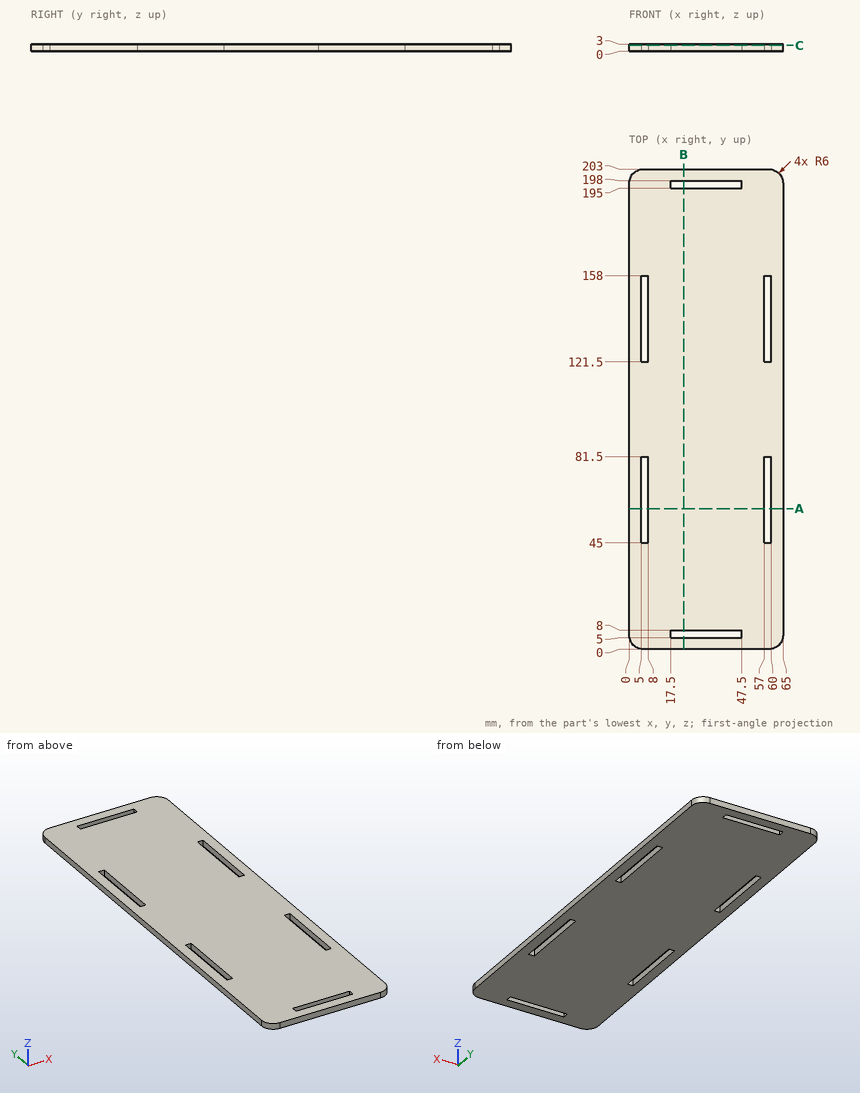
Study the drawing (mm; zero at the part's minimum x, y, z) and answer. Give positions to 0.01 mm unless a question says otherwise; leave off trailing zeros. Write each loop counter-clockwise with the first axis right and the second up, starting at its lowest first coordinate (ties: lowest second). Pieces come first, ordered by that corner, then holes. Notation, with made-up numbers: (14, 70.25) - (24, 70.25) arc R12 cw to (24, 93.25) - close; hole circle Ø8 at (77.5, -39.5). An arc over 180 degrees is marked (long way). Use a Markdown table: item, result.
1. This flat-tipped pin is pushed along its axis until it touches: P1, Ø0.9, axis at y = 59.5, z = 2, coming from the -X side. Where does it stop, or does it pass through?
Values follow:
| item | result |
|---|---|
| P1 | stops at x = 0 |
2. Section C-C on z = 2.45 is taken. Count the separate pieces of the cut face and the enclosed holes in it, plus the area to 3 significant figures.
Values follow:
| item | result |
|---|---|
| separate pieces | 1 |
| enclosed holes | 6 |
| area | 12,500 mm² |
3. Section A-A on y = 59.5 is taken. Write down the section's boundary in (x, z).
Values follow:
| item | result |
|---|---|
| outline | (0, 0) - (5, 0) - (5, 3) - (0, 3) - close; (8, 0) - (57, 0) - (57, 3) - (8, 3) - close; (60, 0) - (65, 0) - (65, 3) - (60, 3) - close |
4. Section B-B on x = 23 is taken. Write down the section's boundary in (y, z).
Values follow:
| item | result |
|---|---|
| outline | (0, 0) - (5, 0) - (5, 3) - (0, 3) - close; (8, 0) - (195, 0) - (195, 3) - (8, 3) - close; (198, 0) - (203, 0) - (203, 3) - (198, 3) - close |
5. Find the intervals of material crossed by probe 1 along Y at (x, z) = (27, 1.1); probe 2 along Y at (x, z) = (6, 2.4); probe 3 along X at (y, z) = (136, 1.5), in increasing order. Write a range as from..to.
Values follow:
| item | result |
|---|---|
| probe 1 | y = 0..5, 8..195, 198..203 |
| probe 2 | y = 0..45, 81.5..121.5, 158..203 |
| probe 3 | x = 0..5, 8..57, 60..65 |
